```python
from build123d import *

# Parameters (mm, degrees)
BASE_FLANGE1_DEPTH           = 1.5
EDGE_FLANGE1_STRIP_W         = 7.4732
EDGE_FLANGE1_STRIP_H         = 1.5
EDGE_FLANGE1_STRIP_CUT_DEPTH = 15
EDGE_FLANGE1_DEPTH           = 15
EDGE_FLANGE2_STRIP_W         = 7.4732
EDGE_FLANGE2_STRIP_H         = 1.5
EDGE_FLANGE2_STRIP_CUT_DEPTH = 15
EDGE_FLANGE2_DEPTH           = 15


# Sheet-metal steps are written as plain solids
with BuildPart() as part:
    # Sketch3 → Base-Flange1 (new body)
    with BuildSketch(Plane.ZY.offset(-75)):
        Polygon((0, 15), (41.5, 15), (41.5, 0), (0, 0), (-4, 0), (-4, 15), align=None)
    extrude(amount=-BASE_FLANGE1_DEPTH)

    # Edge-Flange1 strip (across the edge) → Edge-Flange1 strip cut (cut)
    with BuildSketch(Plane(origin=(75, 0, 41.5), x_dir=(0, 0, -1), z_dir=(0, 1, 0))):
        with Locations((-3, -0.75)):
            Rectangle(EDGE_FLANGE1_STRIP_W, EDGE_FLANGE1_STRIP_H)
    extrude(amount=EDGE_FLANGE1_STRIP_CUT_DEPTH, mode=Mode.SUBTRACT)

    # Edge-Flange1 section (across the edge) → Edge-Flange1 (add)
    with BuildSketch(Plane(origin=(75, 0, 41.5), x_dir=(0, 0, -1), z_dir=(0, 1, 0))):
        with BuildLine():
            Line((-1.5, 0.7366), (-1.5, 91.5))
            Line((-1.5, 91.5), (0, 91.5))
            Line((0, 91.5), (0, 0.7366))
            ThreePointArc((0, 0.7366), (0.215745145, 0.215745145), (0.7366, 0))
            Line((0.7366, 0), (0.7366, -1.5))
            ThreePointArc((0.7366, -1.5), (-0.844915027, -0.844915027), (-1.5, 0.7366))
        make_face()
    extrude(amount=EDGE_FLANGE1_DEPTH)

    # Edge-Flange2 strip (across the edge) → Edge-Flange2 strip cut (cut)
    with BuildSketch(Plane(origin=(-16.5, 0, 41.5), x_dir=(1, 0, 0), z_dir=(0, 1, 0))):
        with Locations((-3, -0.75)):
            Rectangle(EDGE_FLANGE2_STRIP_W, EDGE_FLANGE2_STRIP_H)
    extrude(amount=EDGE_FLANGE2_STRIP_CUT_DEPTH, mode=Mode.SUBTRACT)

    # Edge-Flange2 section (across the edge) → Edge-Flange2 (add)
    with BuildSketch(Plane(origin=(-16.5, 0, 41.5), x_dir=(1, 0, 0), z_dir=(0, 1, 0))):
        with BuildLine():
            Line((-1.5, 0.7366), (-1.5, 45.5))
            Line((-1.5, 45.5), (0, 45.5))
            Line((0, 45.5), (0, 0.7366))
            ThreePointArc((0, 0.7366), (0.215745145, 0.215745145), (0.7366, 0))
            Line((0.7366, 0), (0.7366, -1.5))
            ThreePointArc((0.7366, -1.5), (-0.844915027, -0.844915027), (-1.5, 0.7366))
        make_face()
    extrude(amount=EDGE_FLANGE2_DEPTH)


solid = part.part
```
Geometry check sheet. Reference: the model listing, model coordinates, mm. A direction names the side the tool comes from. Coordinates: 2 decimals unless noted, no trailing zeros. Order: outer loops, then holes, each group sorted by start corner. A loop starts at its lowest first (then second) coordinate and runs counter-clockwise, first axis right, second up. Notation, with made-up numbers: (2, -39) - (52, -39) arc R15 ccw to (52, -35) - close; hole circle Ø7 at (40, -1.75). An arc over 180 degrees is marked (long way). Answer as a JSON object with one key per item and string values. Group by question number.
Item 1: Tool access check on faces 4 (the face through (-16.5, 7, 18)), 5 (the face through (-18, 7, 19)). Record the directions out of +Z, -Z, +X, -X, +Y, -Y that give a thin tool (end or side, any length) a straight path to the whole face; none if there is none.
Item 2: Sectioned sample at B-B, the plane y = 1. Record the cut outline in (x, z).
Item 3: Scan lines: probe 1 along X at (y, z) = (7.75, 40); probe 2 along Z at (x, y) = (8, 8.25). Record each from-to range of solid material in increasing order.
Item 4: Depth check by flat-ended pin: pin 1 Ø7.5 at (x, y) = (47.5, 6.5) entering from -Z. Enter the tip coordinate at first touch or a pass-through.
Item 5: Sectioned sample at C-C, the plane x = 7.5. Record the cut outline in (y, z).
Item 6: Draft check along X on faces 1 (the face through (76.5, 8, 19)), 2 (the face through (30, 7, 43)), 3 (the face through (29, 7, 41.5)). Enter one of: +X half, -X half, draft (parallel to the pull), parting line (faces both ways), or undercut.
Item 7: Sectioned sample at A-A, the plane z = 7. Record the cut outline in (x, y).
Resolved:
{
 "1": {"face 4": "-Z, +Y, -Y", "face 5": "+Z, -Z, -X, +Y, -Y"},
 "2": {"outline": "(-18, -4) - (-16.5, -4) - (-16.5, 40.76) arc R0.74 cw to (-15.76, 41.5) - (74.26, 41.5) arc R0.74 cw to (75, 40.76) - (75, -4) - (76.5, -4) - (76.5, 40.76) arc R2.24 ccw to (74.26, 43) - (-15.76, 43) arc R2.24 ccw to (-18, 40.76) - close"},
 "3": {"probe 1": "-18 to -16.5, 75 to 76.5", "probe 2": "41.5 to 43"},
 "4": {"pin 1": "z = 41.5"},
 "5": {"outline": "(0, 41.5) - (15, 41.5) - (15, 43) - (0, 43) - close"},
 "6": {"face 1": "+X half", "face 2": "draft", "face 3": "undercut"},
 "7": {"outline": "(-18, 0) - (-16.5, 0) - (-16.5, 15) - (-18, 15) - close; (75, 0) - (76.5, 0) - (76.5, 15) - (75, 15) - close"}
}
